Autodesk Inventor part; units mm, degrees
ref_plane "Work Plane1" through (0, 0, 3.81) normal (0, 0, -1) x (-1, 0, 0)
ref_plane "YZ Plane" through (0, 0, 0) normal (1, 0, 0) x (0, 1, 0)
ref_plane "XY Plane" through (0, 0, 0) normal (0, 0, 1) x (1, 0, 0)
sketch "Sketch1" plane through (0, 0, 0) normal (0, 0, 1) x (1, 0, 0)
  circle A0 centre (0, 0) radius 3.81
  dimension "d0" = 7.62
extrude "Extrusion1" add sketch "Sketch1" along normal blind 3.81
hole "Hole1" at (0, 0, 0) direction (0, 0, 1) diameter 5.08 end through all
ref_plane "Work Plane1" through (0, 0, 3.81) normal (0, 0, -1) x (-1, 0, 0)
ref_plane "Work Plane2" through (0, -3.81, 0) normal (0, -1, 0) x (1, 0, 0)
sketch "Sketch2" plane through (0, -3.81, 0) normal (0, -1, 0) x (1, 0, 0)
  point P0 (0, 0)
sketch "Sketch3" plane through (0, -3.81, 0) normal (0, -1, 0) x (1, 0, 0)
  line L0 (-3.81, 3.81) -> (3.81, 3.81)
  line L1 (-3.81, 0) -> (3.81, 0)
  line L2 (0, -0.762) -> (0, 4.572)
  line L3 (0, 3.81) -> (0, 0)
  point P0 (0, 1.905)
  dimension "d15" = 1.905
hole "Hole2" at (0, -3.81, 1.905) direction (0, 1, 0) diameter 1.7018 depth 3.81
equation "\"d12\" = -d1"
properties part number "Jig_Aligner_Sleeve"
Design review of the part built by this model. Coordinates are the model's own, in mm. Coordinates: 2 decimals unless noted, no trailing zeros. Write each loop counter-clockwise with the first axis right and the second up, starting at its lowest first coordinate (ties: lowest second). Pieces come first, ordered by that corner, then holes. Notation, with made-up numbers: (86.25, 66.5) - (118.25, 66.5) arc R21 cw to (118.25, 90.5) - close; hole circle Ø9 at (0, -30). An arc over 180 degrees is marked (long way). Use one line per item in the form item = value.
Q1. Insertion check: pin 1 Ø1 at (y, z) = (2, 2) entering from +X; pin 2 Ø1 at (x, z) = (2, 0.5) entering from +Y. Each pin has a flat end and moves straight along its axis. Give the tip position at first contact, or say it passes through.
Taken from the geometry:
pin_1 = 3.5
pin_2 = 3.5
Q2. The part is to be moulded in two halves that separate along Z. For faces 1 (the flat face through (0, 3, 3.81)), 2 (the cylindrical face through (0.33, -3.09, 1.12)), 3 (the flat face through (0, 3, 0)), say which applies: +Z half, -Z half, draft (parallel to the pull), parting line (faces both ways), or undercut.
Taken from the geometry:
face_1 = +Z half
face_2 = undercut
face_3 = -Z half
Q3. Consider section C-C (z = 3.55). Write out the cut boundary in (x, y).
Taken from the geometry:
outline = circle Ø7.62 at (0, 0); hole circle Ø5.08 at (0, 0)
Q4. For probe 1 along Z at (x, y) = (0, -2.95); probe 2 along Y at (x, z) = (0, 1.1); probe 3 along X at (y, z) = (0.75, 1.6), list the stretches that pass through material, from the lowest coordinate up.
Taken from the geometry:
probe_1 = 0 to 1.05, 2.76 to 3.81
probe_2 = 2.54 to 3.81
probe_3 = -3.74 to -2.43, 2.43 to 3.74
Q5. Consider section D-D (z = 1.7). Write out the cut boundary in (x, y), plus the area to 3 significant figures.
Taken from the geometry:
outline = (-0.83, -3.72) - (-0.83, -2.4) arc R2.54 cw (long way) to (0.83, -2.4) - (0.83, -3.72) arc R3.81 ccw (long way) to start
area = 23.2 mm^2
Q6. Consider section B-B (y = 0.5). Write out the cut boundary in (x, z).
Taken from the geometry:
outline = (-3.78, 0) - (-2.49, 0) - (-2.49, 3.81) - (-3.78, 3.81) - close; (2.49, 0) - (3.78, 0) - (3.78, 3.81) - (2.49, 3.81) - close
Q7. Consider section A-A (x = 0). Write out the cut boundary in (y, z), plus the area to 3 significant figures.
Taken from the geometry:
outline = (-3.81, 0) - (-2.54, 0) - (-2.54, 1.05) - (-3.81, 1.05) - close; (-3.81, 2.76) - (-2.54, 2.76) - (-2.54, 3.81) - (-3.81, 3.81) - close; (2.54, 0) - (3.81, 0) - (3.81, 3.81) - (2.54, 3.81) - close
area = 7.52 mm^2
